```python
from build123d import *

# Parameters (mm, degrees)
SKETCH1_R           = 2.5
BOSS_EXTRUDE1_DEPTH = 15
CUT_EXTRUDE1_START  = -30
SKETCH2_W           = 5
SKETCH2_H           = 40
CUT_EXTRUDE1_DEPTH  = 22.478150705


with BuildPart() as part:
    # Sketch1 → Boss-Extrude1 (new body)
    with BuildSketch(Plane.XY):
        with BuildLine():
            Line((40, 20), (-1.722048604, 4.694097209))
            ThreePointArc((-1.722048604, 4.694097209), (-5, 0), (-1.722048604, -4.694097209))
            Line((-1.722048604, -4.694097209), (40, -20))
            Line((40, -20), (40, 0))
            Line((40, 0), (40, 20))
        make_face()
        Circle(SKETCH1_R, mode=Mode.SUBTRACT)
    extrude(amount=BOSS_EXTRUDE1_DEPTH)

    # Sketch2 → Cut-Extrude1 (cut, through all)
    with BuildSketch(Plane(origin=(40, 0, 0), x_dir=(0, 0, -1), z_dir=(1, 0, 0)).offset(CUT_EXTRUDE1_START)):
        with Locations((-7.5, 0)):
            Rectangle(SKETCH2_W, SKETCH2_H)
    extrude(amount=-CUT_EXTRUDE1_DEPTH, mode=Mode.SUBTRACT)


solid = part.part
```
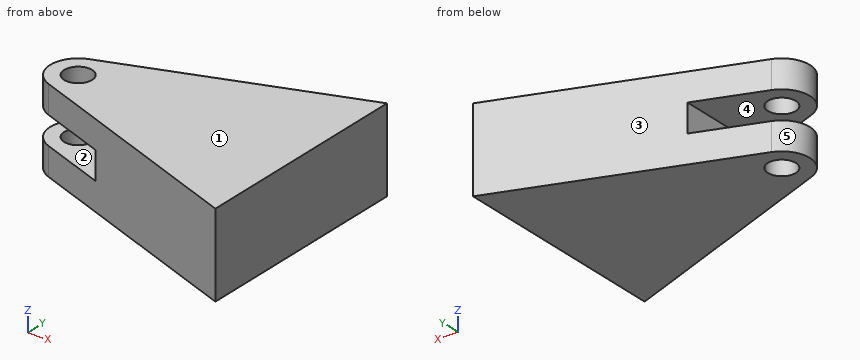
Can you work these out from the model? Positions are in its coordinate system, mm. Face numbers are marked on the shaded views. A direction names the side the tool comes from. Round coordinates to 2 decimals unless told otherwise and drop trailing zeros. Loops run counter-clockwise (first coordinate to the right, second up) from the corner with the lowest first, then second, coordinate; pieces in that order, holes last.
Item 1: Suppose I cut it at B-B, the plane z = 1.5. Write out the boundary of the cut face in (x, y).
Item 2: Will these pins go through, and if not, where does the flat tip stop? pin 1 Ø8 at (x, y) = (0, 0) entering from -Z; pin 2 Ø5 at (x, z) = (5, 5) entering from -Y; pin 3 Ø8 at (x, z) = (32, 5.5) entering from -Y; pin 4 Ø4 at (y, z) = (-1.5, 8.5) entering from -X.
Item 3: Suppose I cut it at D-D, the plane y = 6. Write out the boundary of the cut face in (x, z), then the cut area to 3 significant figures.
Item 4: Which directions (+Z, -Z, +X, -X, +Y, -Y) give clear straight access to the entire face, cutting with the end or side of a thin tool? Please do the marked faces 4 and 5.
Item 5: If we mould it in two halves opening along Z, with no side actions, what happens to the marked faces 1, 2 and 3? For each: +Z half, -Z half, draft (parallel to the pull), parting line (faces both ways), or undercut.
Item 6: Please list where these lines run through material, in increasing order: L1, parallel to X at y = 0, z = 3.1; L2, parallel to Z at x = 4, y = 2.5; L3, parallel to Y at x = 0, z = 1.4.
Item 7: Suppose I cut it at A-A, the plane y = 0. Write out the boundary of the cut face in (x, z).
Item 8: Suppose I cut it at C-C, the plane x = 1.5. Write out the boundary of the cut face in (y, z), then the cut area to 3 significant figures.
Reported:
1. outline: (-1.72, -4.69) - (40, -20) - (40, 20) - (-1.72, 4.69) arc R5 ccw to start; hole circle Ø5 at (0, 0)
2. pin 1: stops at z = 0
2. pin 2: stops at y = -8.08
2. pin 3: stops at y = -18.53
2. pin 4: stops at x = -5
3. outline: (1.84, 0) - (40, 0) - (40, 15) - (1.84, 15) - (1.84, 10) - (10, 10) - (10, 5) - (1.84, 5) - close
3. area: 532 mm2
4. face 4: -X, +Y, -Y
4. face 5: +Z, -Z, -X
5. face 1: +Z half
5. face 2: undercut
5. face 3: draft
6. L1: x = -5 to -2.5, 2.5 to 40
6. L2: z = 0 to 5, 10 to 15
6. L3: y = -5.33 to -2.5, 2.5 to 5.33
7. outline: (-5, 0) - (-2.5, 0) - (-2.5, 5) - (-5, 5) - close; (-5, 10) - (-2.5, 10) - (-2.5, 15) - (-5, 15) - close; (2.5, 0) - (40, 0) - (40, 15) - (2.5, 15) - (2.5, 10) - (10, 10) - (10, 5) - (2.5, 5) - close
8. outline: (-5.88, 0) - (-2, 0) - (-2, 5) - (-5.88, 5) - close; (-5.88, 10) - (-2, 10) - (-2, 15) - (-5.88, 15) - close; (2, 0) - (5.88, 0) - (5.88, 5) - (2, 5) - close; (2, 10) - (5.88, 10) - (5.88, 15) - (2, 15) - close
8. area: 77.5 mm2
